```python
from build123d import *
from build123d.topology import SkipClean

# Parameters (mm, degrees)
SKETCH1_R           = 76.2
SKETCH1_R_2         = 3.175
BOSS_EXTRUDE1_DEPTH = 3.175
SKETCH2_R           = 3.175
CUT_EXTRUDE1_DEPTH  = 108.809835474
CIRPATTERN1_COUNT   = 3
SKETCH3_R           = 3.175
BOSS_EXTRUDE2_DEPTH = 3.175
CIRPATTERN2_COUNT   = 3
FILLET1_R           = 2.54
CUT_EXTRUDE2_DEPTH  = 108.809835619
CIRPATTERN3_COUNT   = 3


with BuildPart() as part:
    # Sketch1 → Boss-Extrude1 (new body)
    with BuildSketch(Plane(origin=(0, 0, 0), x_dir=(1, 0, 0), z_dir=(0, 1, 0))):
        with Locations(Location((0, 0, 0), (0, 0, 270))):
            Circle(SKETCH1_R)
        with Locations(Location((0, 0, 0), (0, 0, 270))):
            Circle(SKETCH1_R_2, mode=Mode.SUBTRACT)
    extrude(amount=BOSS_EXTRUDE1_DEPTH)

    # Sketch2 → Cut-Extrude1 (cut, through all)
    with BuildSketch(Plane(origin=(0, 3.175, 0), x_dir=(1, 0, 0), z_dir=(0, 1, 0))):
        with Locations(Location((69.85, 0, 0), (0, 0, 270))):
            Circle(SKETCH2_R)
    cut_extrude1 = extrude(amount=-CUT_EXTRUDE1_DEPTH, mode=Mode.SUBTRACT)

    # CirPattern1: Cut-Extrude1 ×3 about axis
    cirpattern1_axis = Axis((0, 0, 0), (0, 1, 0))
    for i in range(1, CIRPATTERN1_COUNT):
        add(cut_extrude1.rotate(cirpattern1_axis, i * 360 / CIRPATTERN1_COUNT), mode=Mode.SUBTRACT)

    # Sketch3 → Boss-Extrude2 (add)
    with BuildSketch(Plane(origin=(0, 3.175, 0), x_dir=(1, 0, 0), z_dir=(0, 1, 0))):
        with BuildLine():
            Line((-27.685241282, -54.302244521), (0, -6.35))
            ThreePointArc((0, -6.35), (3.175, 5.499261314), (-5.499261314, -3.175))
            Line((-5.499261314, -3.175), (-33.184502596, -51.127244521))
            ThreePointArc((-33.184502596, -51.127244521), (-38.613147674, -51.709893372), (-42.829980166, -55.178032758))
            ThreePointArc((-42.829980166, -55.178032758), (-62.732354549, -30.719280472), (-69.85, 0))
            Line((-69.85, 0), (-76.2, 0))
            ThreePointArc((-76.2, 0), (-38.1, -65.991135768), (38.1, -65.991135768))
            Line((38.1, -65.991135768), (34.925, -60.491874454))
            ThreePointArc((34.925, -60.491874454), (4.7625, -69.687452915), (-26.370588016, -64.680867246))
            ThreePointArc((-26.370588016, -64.680867246), (-25.47550745, -59.294913492), (-27.685241282, -54.302244521))
        make_face()
        with Locations((-34.925, -60.491874454)):
            Circle(SKETCH3_R, mode=Mode.SUBTRACT)
        Circle(SKETCH3_R, mode=Mode.SUBTRACT)
    boss_extrude2 = extrude(amount=BOSS_EXTRUDE2_DEPTH)

    # CirPattern2: Boss-Extrude2 ×3 about axis
    with SkipClean():  # the faces are left unmerged after this step: merging them gives an invalid solid
        cirpattern2_axis = Axis((0, 0, 0), (0, 1, 0))
        for i in range(1, CIRPATTERN2_COUNT):
            add(boss_extrude2.rotate(cirpattern2_axis, i * 360 / CIRPATTERN2_COUNT))

    # Fillet1
    fillet1_edges = [part.edges().sort_by_distance(p)[0] for p in [
        (0, 4.7625, 6.35),
        (-5.499261314, 4.7625, 3.175),
        (-33.184502596, 4.7625, 51.127244521),
        (-42.829980166, 4.7625, 55.178032758),
        (-26.370588016, 4.7625, 64.680867246),
        (-27.685241282, 4.7625, 54.302244521),
        (-5.499261314, 4.7625, -3.175),
        (5.499261314, 4.7625, -3.175),
        (5.499261314, 4.7625, 3.175),
        (60.869743879, 4.7625, 3.175),
        (69.200568182, 4.7625, 9.502834488),
        (-26.370588016, 4.7625, -64.680867246),
        (69.200568182, 4.7625, -9.502834488),
        (60.869743879, 4.7625, -3.175),
        (0, 4.7625, -6.35),
        (-27.685241282, 4.7625, -54.302244521),
        (-42.829980166, 4.7625, -55.178032758),
        (-33.184502596, 4.7625, -51.127244521),
    ]]
    fillet(fillet1_edges, radius=FILLET1_R)

    # Sketch4 → Cut-Extrude2 (cut, through all)
    with SkipClean():  # the faces are left unmerged after this step: merging them gives an invalid solid
        with BuildSketch(Plane(origin=(0, 3.175, 0), x_dir=(1, 0, 0), z_dir=(0, 1, 0))):
            with BuildLine():
                Line((-6.154438838, 4.30980076), (-32.361839489, 49.702350221))
                ThreePointArc((-32.361839489, 49.702350221), (-33.324824736, 50.650936578), (-34.638061064, 50.971197428))
                ThreePointArc((-34.638061064, 50.971197428), (-38.278807741, 51.576853499), (-41.416002253, 53.521041308))
                ThreePointArc((-41.416002253, 53.521041308), (-43.078433965, 54.20122857), (-44.775122458, 53.611667656))
                ThreePointArc((-44.775122458, 53.611667656), (-69.85, 0), (-44.775122458, -53.611667656))
                ThreePointArc((-44.775122458, -53.611667656), (-43.078433965, -54.20122857), (-41.416002253, -53.521041308))
                ThreePointArc((-41.416002253, -53.521041308), (-38.278807741, -51.576853499), (-34.638061064, -50.971197428))
                ThreePointArc((-34.638061064, -50.971197428), (-33.324824736, -50.650936578), (-32.361839489, -49.702350221))
                Line((-32.361839489, -49.702350221), (-6.154438838, -4.30980076))
                ThreePointArc((-6.154438838, -4.30980076), (-5.823818881, -3.261291188), (-5.96724526, -2.171286257))
                ThreePointArc((-5.96724526, -2.171286257), (-6.35, 0), (-5.96724526, 2.171286257))
                ThreePointArc((-5.96724526, 2.171286257), (-5.823818881, 3.261291188), (-6.154438838, 4.30980076))
            make_face()
        cut_extrude2 = extrude(amount=-CUT_EXTRUDE2_DEPTH, mode=Mode.SUBTRACT)

    # CirPattern3: Cut-Extrude2 ×3 about axis
    with SkipClean():  # the faces are left unmerged after this step: merging them gives an invalid solid
        cirpattern3_axis = Axis((0, 3.175, 0), (0, -1, 0))
        for i in range(1, CIRPATTERN3_COUNT):
            add(cut_extrude2.rotate(cirpattern3_axis, i * 360 / CIRPATTERN3_COUNT), mode=Mode.SUBTRACT)


solid = part.part
```
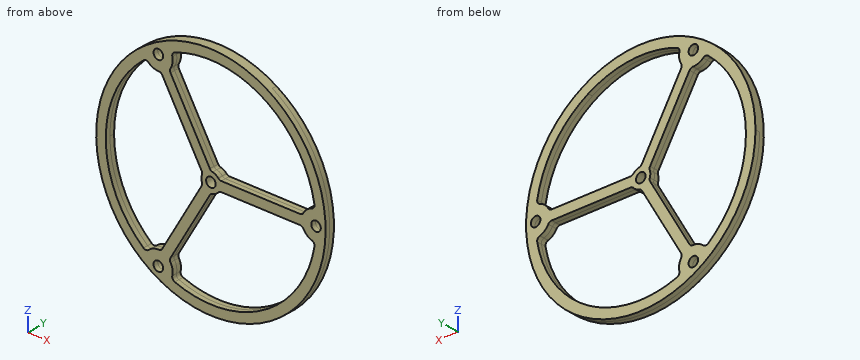
Read the model definition and answer for the solid it produces. Units are mm, in the model's axes. Give positions to 0.01 mm unless a question says otherwise; leave off trailing zeros. Order: outer loops, then holes, each group sorted by start corner. A loop starts at its lowest first (then second) coordinate and runs counter-clockwise, first axis right, second up.
(1) Find section D-D (y = 1). Give the number of separate pieces and of enclosed holes in the cut face, plus the area to 3 significant figures.
(2) Find section C-C (z = -33). Give the vertices of the cut face in (x, y) (3 decimals).
(3) Find section A-A (x = 47.5). Give the vertices of the cut face in (y, z) (3 decimals), plus the area to 3 significant figures.
(4) Given pin 1 (2.5 mm diameter, centred on x = 43.5, y = 5, fed in from +Z); pin 2 (2 mm diameter, centred on x = -25.5, y = 5, fed in from -Z); pin 3 (3.5 mm diameter, centred on x = 34.5, y = 1.5, fed in from +Z), each flat-ended and moving along its own axis, determine where each tip first touches the part or whether it passes through.
(5) Straight lines are drawn through the part: L1, parallel to Z at x = 64.5, y = 2.5; L2, parallel to X at y = 0.75, z = 16; L3, parallel to Z at x = 25, y = 3 (3 decimals). For each, find the intervals that lie inside material, in ascending order.
Result sheet:
1. separate pieces: 1
1. enclosed holes: 7
1. area: 4,380 mm2
2. outline: (-68.684, 0) - (-61.563, 0) - (-61.563, 6.35) - (-68.684, 6.35) - close; (-22.719, 0) - (-15.386, 0) - (-15.386, 6.35) - (-22.719, 6.35) - close; (61.563, 0) - (68.684, 0) - (68.684, 6.35) - (61.563, 6.35) - close
3. outline: (0, -59.583) - (6.35, -59.583) - (6.35, -51.213) - (0, -51.213) - close; (0, -3.175) - (6.35, -3.175) - (6.35, 3.175) - (0, 3.175) - close; (0, 51.213) - (6.35, 51.213) - (6.35, 59.583) - (0, 59.583) - close
3. area: 147 mm2
4. pin 1: stops at z = 63.41
4. pin 2: stops at z = -72.15
4. pin 3: stops at z = 68.8
5. L1: z = -40.57 to -26.81, -7.88 to 7.88, 26.81 to 40.57
5. L2: x = -74.5 to -67.99, -12.9 to -5.57, 67.99 to 74.5
5. L3: z = -71.982 to -65.223, -3.175 to 3.175, 65.223 to 71.982
